Geometry: final body of the model. Coordinates: model frame, mm. Face numbers are marked on the shaded views. A direction names the side the tool comes from. Round coordinates to 2 decimals unless told otherwise and drop trailing zeros. Write each loop counter-clockwise with the first axis right and the second up, starting at its lowest first coordinate (ties: lowest second). Pieces come first, ordered by that corner, then holes. Notation, with made-up numbers: (53.5, 41.5) - (108.5, 41.5) arc R24 ccw to (108.5, 67.5) - close; hole circle Ø11 at (52.25, 78.5). An arc over 180 degrees is marked (long way). Write each question's results on one line, items separated by ' | '.
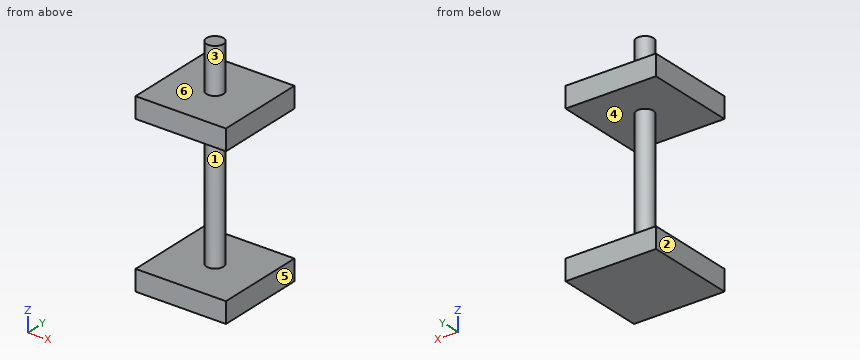
from build123d import *

# Parameters (mm, degrees)
F0_W     = 50.8
F0_H     = 50.8
F1_DEPTH = 11.5824
F2_R     = 4.7625
F3_DEPTH = 76.2
F4_W     = 50.8
F4_H     = 50.8
F4_R     = 4.7625
F5_DEPTH = 11.5824
F6_R     = 4.7625
F7_DEPTH = 25.4


with BuildPart() as f1:
    # F0 (on Top) → F1 (new body)
    with BuildSketch(Plane.XY):
        Rectangle(F0_W, F0_H)
    extrude(amount=F1_DEPTH)

    # F2 (on face) → F3 (join)
    with BuildSketch(Plane.XY.offset(11.5824)):
        Circle(F2_R)
    extrude(amount=F3_DEPTH)

    # F4 (on face) → F5 (join)
    with BuildSketch(Plane.XY.offset(87.7824)):
        Rectangle(F4_W, F4_H)
        Circle(F4_R, mode=Mode.SUBTRACT)
        Circle(F4_R)
    extrude(amount=F5_DEPTH)

    # F6 (on face) → F7 (join)
    with BuildSketch(Plane.XY.offset(99.3648)):
        Circle(F6_R)
    extrude(amount=F7_DEPTH)


solid = f1.part
Q1. Access query for the marked faces 1, 2 and 3. Directions: +Z, -Z, +X, -X, +Y, -Y. A direction counts if a zero-diameter tool reaches every point of the face in a straight line with its end or side. Return the directions, or none.
Answer block:
face 1: none | face 2: +Z, -Z, -X, +Y, -Y | face 3: +Z
Q2. Mould query, pull axis Z, two halves, no side actions, for the marked faces 4, 5 and 6. Classes: pulls with the +Z half, pulls with the -Z half, needs draft (parallel to the pull), parting line crosses it, or undercut.
Answer block:
face 4: undercut | face 5: needs draft | face 6: pulls with the +Z half
Q3. Pin query (flat end, axial travel): pin 1 (10 mm diameter, centred on x = 4.5, y = 16.5, fed in from +Z); pin 2 (3 mm diameter, centred on x = 7.5, z = 101.5, fed in from -Y). Return the tip coordinate at first contact, or that it passes through.
Answer block:
pin 1: z = 99.36 | pin 2: through
Q4. Section query C-C, the plane y = 0. Return loops of the section in (x, z), plus the area to 3 significant figures.
Answer block:
outline: (-25.4, 0) - (25.4, 0) - (25.4, 11.58) - (4.76, 11.58) - (4.76, 87.78) - (25.4, 87.78) - (25.4, 99.36) - (4.76, 99.36) - (4.76, 124.76) - (-4.76, 124.76) - (-4.76, 99.36) - (-25.4, 99.36) - (-25.4, 87.78) - (-4.76, 87.78) - (-4.76, 11.58) - (-25.4, 11.58) - close | area: 2,140 mm2
Q5. Ray query, line 1 along Z through (x, y) = (7, 1.5). Return the intervals inside material, ascending.
Answer block:
line 1: 0 to 11.58, 87.78 to 99.36
Q6. Section query A-A, the plane y = -12.5. Return loops of the section in (x, z).
Answer block:
outline: (-25.4, 0) - (25.4, 0) - (25.4, 11.58) - (-25.4, 11.58) - close; (-25.4, 87.78) - (25.4, 87.78) - (25.4, 99.36) - (-25.4, 99.36) - close
